Part model, mm, in its own coordinate system. A direction names the side the tool comes from. Give positions to 0.01 mm unless a question says otherwise; leave off trailing zeros. Order: outer loops, then holes, each group sorted by start corner. A loop starts at its lowest first (then second) coordinate and runs counter-clockwise, first axis right, second up. Notation, with made-up numbers: (51.5, 59.5) - (81.5, 59.5) arc R22 ccw to (81.5, 86.5) - close; hole circle Ø9 at (-24.75, 0). An arc over 180 degrees is marked (long way). Use one line per item in the form item = value. Start each with the question number.
1. Pin check, flat tips, straight feed: P1, Ø7.5, axis at x = 39.5, y = 28.5, coming from the +Z side; P2, Ø1.5, axis at x = 45, y = 25, coming from the -Z side; P3, Ø10, axis at y = 17, z = -13, coming from the +X side; P4, Ø7.5, axis at x = 27, y = 26, coming from the -Z side. Stop position of each tip, or through.
2. Pull direction X, two halves, no side cores. Call faces 1 (the face through (32, 21, 15.5)), 2 (the face through (25, 18, 0)), 3 (the face through (-5, 20, -10)): +X half, -X half, draft (parallel to the pull), parting line (faces both ways), or undercut.
3. Tool access for faces 4 (the face through (-7, 21, -20)), 5 (the face through (33, 18, 17)), 6 (the face through (16, 19, 4)), 7 (the face through (33, 18, 2)): list every direction of +Z, -Z, +X, -X, +Y, -Y with a clear straight run to the whole face (end or side of a thin tool).
4. Band-saw the part on A-A, the plane x = 7. List the corners of the cut face in (y, z), plus the area to 4 significant figures.
5. Band-saw the part on C-C, the plane y = 20. State how many separate pieces and enclosed holes the cut face has, plus the area to 3 significant figures.
6. Band-saw the part on B-B, the plane z = -7.5. List the corners of the cut face in (x, y), plus the area to 4 significant figures.
7. Drill centre lines: line 1 (Z direction, x = 35, y = 20); line 2 (Z direction, x = 7, y = 6.3); line 3 (X direction, y = 6, z = -7.5). Where is each one in solid material? Low to high.
8. Band-saw the part on D-D, the plane z = 2.5. List the corners of the cut face in (x, y), plus the area to 3 significant figures.
from build123d import *

# Parameters (mm, degrees)
SKETCH1_W            = 66
SKETCH1_H            = 33
BOSS_EXTRUDE1_DEPTH  = 4
CUT_EXTRUDE1_DEPTH   = 5
BOSS_EXTRUDE2_DEPTH  = 20
BOSS_EXTRUDE3_DEPTH  = 1.3
BOSS_EXTRUDE4_DEPTH  = 1.3
BOSS_EXTRUDE5_DEPTH  = 1.3
BOSS_EXTRUDE6_DEPTH  = 1.3
SKETCH11_W           = 66
SKETCH11_H           = 8
CUT_EXTRUDE4_DEPTH   = 10
SKETCH13_W           = 4
SKETCH13_H           = 25
BOSS_EXTRUDE7_DEPTH  = 9
SKETCH14_W           = 4
SKETCH14_H           = 25
BOSS_EXTRUDE8_DEPTH  = 8
SKETCH16_R           = 1.75
CUT_EXTRUDE5_DEPTH   = 12
SKETCH17_R           = 1.75
CUT_EXTRUDE8_DEPTH   = 12
SKETCH18_W           = 4
SKETCH18_H           = 25
CUT_EXTRUDE9_DEPTH   = 3
SKETCH19_W           = 4
SKETCH19_H           = 25
BOSS_EXTRUDE10_DEPTH = 4
SKETCH20_W           = 4
SKETCH20_H           = 25
BOSS_EXTRUDE11_DEPTH = 20
SKETCH21_R           = 1.75
CUT_EXTRUDE10_DEPTH  = 20
SKETCH22_W           = 20
SKETCH22_H           = 25
CUT_EXTRUDE11_DEPTH  = 20
SKETCH23_W           = 4
SKETCH23_H           = 25
BOSS_EXTRUDE12_DEPTH = 20
SKETCH24_R           = 1.75
CUT_EXTRUDE12_DEPTH  = 85
SKETCH25_W           = 25
SKETCH25_H           = 26
BOSS_EXTRUDE13_DEPTH = 3
SKETCH26_R           = 1.75
CUT_EXTRUDE13_DEPTH  = 29
SKETCH27_W           = 20
SKETCH27_H           = 25
CUT_EXTRUDE14_DEPTH  = 27


with BuildPart() as part:
    # Sketch1 → Boss-Extrude1 (new body)
    with BuildSketch(Plane.XY):
        with Locations((33, 16.5)):
            Rectangle(SKETCH1_W, SKETCH1_H)
    extrude(amount=BOSS_EXTRUDE1_DEPTH)

    # Sketch2 → Cut-Extrude1 (cut, through all)
    with BuildSketch(Plane.XY.offset(4)):
        with BuildLine():
            Line((18, 33), (48, 33))
            ThreePointArc((48, 33), (33, 18), (18, 33))
        make_face()
    extrude(amount=-CUT_EXTRUDE1_DEPTH, mode=Mode.SUBTRACT)

    # Sketch3 → Boss-Extrude2 (add)
    with BuildSketch(Plane.XY.offset(4)):
        with BuildLine():
            Line((18, 33), (15.5, 33))
            ThreePointArc((15.5, 33), (33, 15.5), (50.5, 33))
            Line((50.5, 33), (48, 33))
            ThreePointArc((48, 33), (33, 18), (18, 33))
        make_face()
    extrude(amount=BOSS_EXTRUDE2_DEPTH)

    # Sketch5 → Boss-Extrude3 (add)
    with BuildSketch(Plane.XY.offset(4.6)):
        with BuildLine():
            Line((18, 33), (21.25, 33))
            ThreePointArc((21.25, 33), (33, 21.25), (44.75, 33))
            Line((44.75, 33), (48, 33))
            ThreePointArc((48, 33), (33, 18), (18, 33))
        make_face()
    extrude(amount=BOSS_EXTRUDE3_DEPTH)

    # Sketch6 → Boss-Extrude4 (add)
    with BuildSketch(Plane.XY.offset(9.4)):
        with BuildLine():
            Line((18, 33), (21.25, 33))
            ThreePointArc((21.25, 33), (33, 21.25), (44.75, 33))
            Line((44.75, 33), (48, 33))
            ThreePointArc((48, 33), (33, 18), (18, 33))
        make_face()
    extrude(amount=BOSS_EXTRUDE4_DEPTH)

    # Sketch7 → Boss-Extrude5 (add)
    with BuildSketch(Plane.XY.offset(14.2)):
        with BuildLine():
            Line((18, 33), (21.25, 33))
            ThreePointArc((21.25, 33), (33, 21.25), (44.75, 33))
            Line((44.75, 33), (48, 33))
            ThreePointArc((48, 33), (33, 18), (18, 33))
        make_face()
    extrude(amount=BOSS_EXTRUDE5_DEPTH)

    # Sketch8 → Boss-Extrude6 (add)
    with BuildSketch(Plane.XY.offset(19)):
        with BuildLine():
            Line((18, 33), (21.25, 33))
            ThreePointArc((21.25, 33), (33, 21.25), (44.75, 33))
            Line((44.75, 33), (48, 33))
            ThreePointArc((48, 33), (33, 18), (18, 33))
        make_face()
    extrude(amount=BOSS_EXTRUDE6_DEPTH)

    # Sketch11 → Cut-Extrude4 (cut)
    with BuildSketch(Plane.XY.offset(4)):
        with Locations((33, 4)):
            Rectangle(SKETCH11_W, SKETCH11_H)
    extrude(amount=-CUT_EXTRUDE4_DEPTH, mode=Mode.SUBTRACT)

    # Sketch13 → Boss-Extrude7 (add)
    with BuildSketch(Plane.ZY):
        with Locations((2, 20.5)):
            Rectangle(SKETCH13_W, SKETCH13_H)
    extrude(amount=BOSS_EXTRUDE7_DEPTH)

    # Sketch14 → Boss-Extrude8 (add)
    with BuildSketch(Plane(origin=(66, 0, 0), x_dir=(0, 0, -1), z_dir=(1, 0, 0))):
        with Locations((-2, 20.5)):
            Rectangle(SKETCH14_W, SKETCH14_H)
    extrude(amount=BOSS_EXTRUDE8_DEPTH)

    # Sketch16 → Cut-Extrude5 (cut)
    with BuildSketch(Plane(origin=(74, 0, 0), x_dir=(0, 0, -1), z_dir=(1, 0, 0))):
        with Locations((14, 13)):
            Circle(SKETCH16_R)
    extrude(amount=-CUT_EXTRUDE5_DEPTH, mode=Mode.SUBTRACT)

    # Sketch17 → Cut-Extrude8 (cut)
    with BuildSketch(Plane.XY.offset(4)):
        with Locations((59, 13)):
            Circle(SKETCH17_R)
    extrude(amount=-CUT_EXTRUDE8_DEPTH, mode=Mode.SUBTRACT)

    # Sketch18 → Cut-Extrude9 (cut)
    with BuildSketch(Plane(origin=(74, 0, 0), x_dir=(0, 0, -1), z_dir=(1, 0, 0))):
        with Locations((-2, 20.5)):
            Rectangle(SKETCH18_W, SKETCH18_H)
    extrude(amount=-CUT_EXTRUDE9_DEPTH, mode=Mode.SUBTRACT)

    # Sketch19 → Boss-Extrude10 (add)
    with BuildSketch(Plane(origin=(71, 0, 0), x_dir=(0, 0, -1), z_dir=(1, 0, 0))):
        with Locations((-2, 20.5)):
            Rectangle(SKETCH19_W, SKETCH19_H)
    extrude(amount=BOSS_EXTRUDE10_DEPTH)

    # Sketch20 → Boss-Extrude11 (add)
    with BuildSketch(Plane(origin=(0, 0, 0), x_dir=(-1, 0, 0), z_dir=(0, 0, -1))):
        with Locations((-73, 20.5)):
            Rectangle(SKETCH20_W, SKETCH20_H)
    extrude(amount=BOSS_EXTRUDE11_DEPTH)

    # Sketch21 → Cut-Extrude10 (cut)
    with BuildSketch(Plane(origin=(75, 0, 0), x_dir=(0, 0, -1), z_dir=(1, 0, 0))):
        with Locations((14, 13)):
            Circle(SKETCH21_R)
    extrude(amount=-CUT_EXTRUDE10_DEPTH, mode=Mode.SUBTRACT)

    # Sketch22 → Cut-Extrude11 (cut)
    with BuildSketch(Plane(origin=(75, 0, 0), x_dir=(0, 0, -1), z_dir=(1, 0, 0))):
        with Locations((10, 20.5)):
            Rectangle(SKETCH22_W, SKETCH22_H)
    extrude(amount=-CUT_EXTRUDE11_DEPTH, mode=Mode.SUBTRACT)

    # Sketch23 → Boss-Extrude12 (add)
    with BuildSketch(Plane(origin=(0, 0, 0), x_dir=(-1, 0, 0), z_dir=(0, 0, -1))):
        with Locations((7, 20.5)):
            Rectangle(SKETCH23_W, SKETCH23_H)
    extrude(amount=BOSS_EXTRUDE12_DEPTH)

    # Sketch24 → Cut-Extrude12 (cut, through all)
    with BuildSketch(Plane.ZY.offset(9)):
        with Locations((-7.5, 20)):
            Circle(SKETCH24_R)
    extrude(amount=-CUT_EXTRUDE12_DEPTH, mode=Mode.SUBTRACT)

    # Sketch25 → Boss-Extrude13 (add)
    with BuildSketch(Plane(origin=(0, 8, 0), x_dir=(-1, 0, 0), z_dir=(0, -1, 0))):
        with Locations((-3.5, 9)):
            Rectangle(SKETCH25_W, SKETCH25_H)
    extrude(amount=BOSS_EXTRUDE13_DEPTH)

    # Sketch26 → Cut-Extrude13 (cut, through all)
    with BuildSketch(Plane(origin=(0, 5, 0), x_dir=(-1, 0, 0), z_dir=(0, -1, 0))):
        with Locations((-7, 7.5)):
            Circle(SKETCH26_R)
    extrude(amount=-CUT_EXTRUDE13_DEPTH, mode=Mode.SUBTRACT)

    # Sketch27 → Cut-Extrude14 (cut, through all)
    with BuildSketch(Plane.XY.offset(4)):
        with Locations((65, 20.5)):
            Rectangle(SKETCH27_W, SKETCH27_H)
    extrude(amount=-CUT_EXTRUDE14_DEPTH, mode=Mode.SUBTRACT)


solid = part.part
From the geometry:
q1.P1 = through
q1.P2 = 0
q1.P3 = -5
q1.P4 = 4.6
q2.face_1 = undercut
q2.face_2 = draft
q2.face_3 = +X half
q3.face_4 = -Z, +X, -X, +Y
q3.face_5 = +Y
q3.face_6 = +Z, -Y
q3.face_7 = -Z, +Y
q4.outline = (5, -22) - (8, -22) - (8, -9.25) - (5, -9.25) - close; (5, -5.75) - (8, -5.75) - (8, 0) - (33, 0) - (33, 4) - (5, 4) - close
q4.area = 167.5 mm²
q5.separate_pieces = 2
q5.enclosed_holes = 3
q5.area = 509 mm²
q6.outline = (-9, 5) - (5.25, 5) - (5.25, 8) - (-5, 8) - (-5, 18.25) - (-9, 18.25) - close; (-9, 21.75) - (-5, 21.75) - (-5, 33) - (-9, 33) - close; (8.75, 5) - (16, 5) - (16, 8) - (8.75, 8) - close
q6.area = 150.5 mm²
q7.line_1 = 4.6 to 5.9, 9.4 to 10.7, 14.2 to 15.5, 19 to 20.3
q7.line_2 = -22 to -9.25, -5.75 to 4
q7.line_3 = -9 to 5.25, 8.75 to 16
q8.outline = (-9, 5) - (16, 5) - (16, 8) - (55, 8) - (55, 33) - (48, 33) arc R15 cw to (18, 33) - (-9, 33) - close
q8.area = 1,320 mm²
